Read the model definition and answer for the solid it produces. Units are mm, in the model's axes. Face numbers are marked on the shaded views. A direction names the side the tool comes from. Coordinates: 2 decimals unless noted, no trailing zeros. Order: outer loops, then holes, each group sorted by start corner. A loop starts at its lowest first (then second) coordinate and runs counter-clockwise, first axis right, second up. Notation, with made-up numbers: M 53,-38.75 L 67,-38.75 A33 ccw 67,-6.75 Z; hole C -11.75,-9 d3. An arc over 180 degrees is marked long. Use a Markdown table: item, result. Add a question column.
1) Find section A-A on x = 62. Write down the section's boundary in (y, z), plus the area to 3 significant figures.
2) For the marked faces 1 and 2, determine the directions among +Z, -Z, +X, -X, +Y, -Y from which every point of the face is accessible in a straight line to the end or side of a thin tool.
3) Find section B-B on y = 5. Count the separate pieces of the cut face and the enclosed holes in it, plus the area to 3 significant figures.
4) Find section D-D on y = 69.5. Write down the section's boundary in (x, z).
5) Find the intervals of material crossed by probe 1 along Y at (x, z) = (53, 17); probe 2 along X at (y, z) = (6, 10.5); probe 3 along Z at (x, y) = (73, 27.5), in increasing order. Write a range as [from, to].
6) Find section C-C on z = 126. Write down the section's boundary in (x, y), plus the area to 3 significant figures.
7) Each of these flat-tipped pins is pushed along its axis until it touches: pin 1 Ø6 at (x, z) = (59, 127) entering from +Y; pin 2 Ø5.5 at (y, z) = (22, -18.5) entering from +X; pin 3 Ø15.5 at (x, z) = (88, 159) entering from +Y. Where does it stop, or does it pass through?
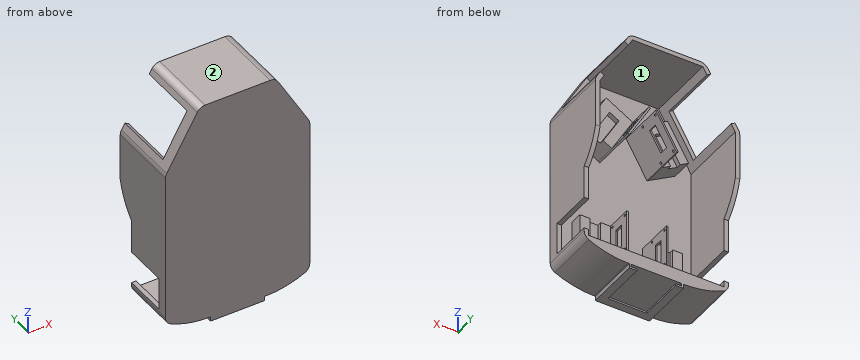
from build123d import *

# Parameters (mm, degrees)
BOSS_EXTRUDE1_DEPTH  = 80
BOSS_EXTRUDE2_DEPTH  = 2
SKETCH9_W            = 34
SKETCH9_H            = 46.5
BOSS_EXTRUDE3_DEPTH  = 13.75
SKETCH13_W           = 46.5
SKETCH13_H           = 42.25
BOSS_EXTRUDE7_DEPTH  = 2
SKETCH14_R           = 1.25
SKETCH14_W           = 25
SKETCH14_H           = 10
CUT_EXTRUDE1_DEPTH   = 2
SKETCH15_W           = 12
SKETCH15_H           = 35
CUT_EXTRUDE2_DEPTH   = 5
CUT_EXTRUDE3_DEPTH   = 298.215141228
FILLET5_R            = 10
SKETCH16_W           = 36
SKETCH16_H           = 48
CUT_EXTRUDE4_DEPTH   = 5
BOSS_EXTRUDE16_DEPTH = 23.75
SKETCH39_W           = 46.5
SKETCH39_H           = 52.25
BOSS_EXTRUDE17_DEPTH = 2
SKETCH40_R           = 1.25
SKETCH40_W           = 25
SKETCH40_H           = 10
CUT_EXTRUDE10_DEPTH  = 2
CUT_EXTRUDE11_DEPTH  = 5
SKETCH43_W           = 54
SKETCH43_H           = 67
CUT_EXTRUDE12_DEPTH  = 5
SKETCH44_W           = 150
SKETCH44_H           = 10
BOSS_EXTRUDE18_DEPTH = 60
SKETCH45_W           = 60
SKETCH45_H           = 60
BOSS_EXTRUDE19_DEPTH = 5
FILLET8_R            = 10
FILLET9_R            = 100
CUT_EXTRUDE13_DEPTH  = 51
SKETCH48_W           = 56
SKETCH48_H           = 3
CUT_EXTRUDE14_DEPTH  = 7


with BuildPart() as part:
    # Sketch1 → Boss-Extrude1 (new body)
    with BuildSketch(Plane(origin=(0, 0, 0), x_dir=(1, 0, 0), z_dir=(0, 1, 0))):
        Polygon((-5, 5), (-5, -171.339745962), (33.113248654, -237.353829072), (116.886751346, -237.353829072), (155, -171.339745962), (155, 5), align=None)
        Polygon((0, 0), (0, -170), (36, -232.353829072), (114, -232.353829072), (150, -170), (150, 0), align=None, mode=Mode.SUBTRACT)
    extrude(amount=BOSS_EXTRUDE1_DEPTH)



with BuildPart() as body_2:
    # Sketch8 → Boss-Extrude2 (new body)
    with BuildSketch(Plane.XZ):
        Polygon((0, 0), (0, 170), (36, 232.353829072), (114, 232.353829072), (150, 170), (150, 0), align=None)
    extrude(amount=-BOSS_EXTRUDE2_DEPTH)


with BuildPart() as part_1:
    add(part.part)

    add(body_2.part)  # Boss-Extrude3 merges body 2
    # Sketch9 → Boss-Extrude3 (add)
    with BuildSketch(Plane(origin=(0, 2, 0), x_dir=(1, 0, 0), z_dir=(0, 1, 0))):
        with Locations((115, -37)):
            Rectangle(SKETCH9_W, SKETCH9_H)
    boss_extrude3 = extrude(amount=BOSS_EXTRUDE3_DEPTH)

    # Sketch13 → Boss-Extrude7 (add)
    with BuildSketch(Plane.ZY.offset(-98)):
        with Locations((37, 23.125)):
            Rectangle(SKETCH13_W, SKETCH13_H)
    boss_extrude7 = extrude(amount=BOSS_EXTRUDE7_DEPTH)

    # Sketch14 → Cut-Extrude1 (cut)
    with BuildSketch(Plane.ZY.offset(-96)):
        with Locations((17, 41)):
            Circle(SKETCH14_R)
        with Locations((57, 41)):
            Circle(SKETCH14_R)
        with Locations(Location((57, 19, 0), (0, 0, 180))):
            Circle(SKETCH14_R)
        with Locations(Location((17, 19, 0), (0, 0, 180))):
            Circle(SKETCH14_R)
        with Locations((37, 30)):
            Rectangle(SKETCH14_W, SKETCH14_H)
    cut_extrude1 = extrude(amount=-CUT_EXTRUDE1_DEPTH, mode=Mode.SUBTRACT)

    # Sketch15 → Cut-Extrude2 (cut)
    with BuildSketch(Plane(origin=(0, 15.75, 0), x_dir=(1, 0, 0), z_dir=(0, 1, 0))):
        with Locations((115, -42.75)):
            Rectangle(SKETCH15_W, SKETCH15_H)
    cut_extrude2 = extrude(amount=-CUT_EXTRUDE2_DEPTH, mode=Mode.SUBTRACT)

    # Sketch17 → Cut-Extrude3 (cut, through all)
    with BuildSketch(Plane(origin=(155, 0, 0), x_dir=(0, 0, -1), z_dir=(1, 0, 0))):
        with BuildLine():
            Line((5, 60), (-80, 60))
            ThreePointArc((-80, 60), (-96.561006469, 72.526691771), (-115.934560766, 80))
            Line((-115.934560766, 80), (5, 80))
            Line((5, 80), (5, 60))
        make_face()
    extrude(amount=-CUT_EXTRUDE3_DEPTH, mode=Mode.SUBTRACT)

    # Fillet5
    fillet5_edges = [part_1.edges().sort_by_distance(p)[0] for p in [
        (-5, 40, 171.339745962),
        (33.113248654, 40, 237.353829072),
        (116.886751346, 40, 237.353829072),
        (155, 40, 171.339745962),
    ]]
    fillet(fillet5_edges, radius=FILLET5_R)

    # Sketch16 → Cut-Extrude4 (cut)
    with BuildSketch(Plane.ZY.offset(-150)):
        with Locations((25, 36)):
            Rectangle(SKETCH16_W, SKETCH16_H)
    cut_extrude4 = extrude(amount=-CUT_EXTRUDE4_DEPTH, mode=Mode.SUBTRACT)

    # Sketch38 → Boss-Extrude16 (add)
    with BuildSketch(Plane(origin=(0, 2, 0), x_dir=(1, 0, 0), z_dir=(0, 1, 0))):
        Polygon((109.054491924, -200.919700329), (132.304491924, -160.649519053), (102.859628196, -143.649519053), (79.609628196, -183.919700329), align=None)
    boss_extrude16 = extrude(amount=BOSS_EXTRUDE16_DEPTH)

    # Sketch39 → Boss-Extrude17 (add)
    with BuildSketch(Plane(origin=(139.346787517, 0, 80.451905284), x_dir=(-0.4999999999999941, 0, 0.866025403784442), z_dir=(-0.8660254037844421, 0, -0.49999999999999417))):
        with Locations((96.224318643, 28.125)):
            Rectangle(SKETCH39_W, SKETCH39_H)
    boss_extrude17 = extrude(amount=BOSS_EXTRUDE17_DEPTH)

    # Sketch40 → Cut-Extrude10 (cut)
    with BuildSketch(Plane(origin=(137.61473671, 0, 79.451905284), x_dir=(-0.4999999999999936, 0, 0.8660254037844424), z_dir=(-0.8660254037844424, 0, -0.4999999999999936))):
        with Locations((76.224318643, 51)):
            Circle(SKETCH40_R)
        with Locations(Location((116.224318643, 51, 0), (0, 0, 180))):
            Circle(SKETCH40_R)
        with Locations((116.224318643, 29)):
            Circle(SKETCH40_R)
        with Locations(Location((76.224318643, 29, 0), (0, 0, 180))):
            Circle(SKETCH40_R)
        with Locations((96.224318643, 40)):
            Rectangle(SKETCH40_W, SKETCH40_H)
    cut_extrude10 = extrude(amount=-CUT_EXTRUDE10_DEPTH, mode=Mode.SUBTRACT)

    # Sketch42 → Cut-Extrude11 (cut)
    with BuildSketch(Plane(origin=(0, 25.75, 0), x_dir=(1, 0, 0), z_dir=(0, 1, 0))):
        Polygon((105.278212483, -185.460408185), (122.778212483, -155.149519053), (112.385907637, -149.149519053), (94.885907637, -179.460408185), align=None)
    cut_extrude11 = extrude(amount=-CUT_EXTRUDE11_DEPTH, mode=Mode.SUBTRACT)

    # Sketch43 → Cut-Extrude12 (cut)
    with BuildSketch(Plane(origin=(186.112159322, 0, 107.451905284), x_dir=(-0.5000000000000009, 0, 0.8660254037844383), z_dir=(-0.8660254037844382, 0, -0.5000000000000008))):
        with Locations((108.224318643, 46.5)):
            Rectangle(SKETCH43_W, SKETCH43_H)
    cut_extrude12 = extrude(amount=-CUT_EXTRUDE12_DEPTH, mode=Mode.SUBTRACT)

    # Mirror1: Boss-Extrude3, Boss-Extrude7, Cut-Extrude1, Cut-Extrude2, Cut-Extrude4, Boss-Extrude16, Boss-Extrude17, Cut-Extrude10, Cut-Extrude11, Cut-Extrude12 across plane
    add(boss_extrude3.mirror(Plane.ZY.offset(-75)))
    add(boss_extrude7.mirror(Plane.ZY.offset(-75)))
    add(cut_extrude1.mirror(Plane.ZY.offset(-75)), mode=Mode.SUBTRACT)
    add(cut_extrude2.mirror(Plane.ZY.offset(-75)), mode=Mode.SUBTRACT)
    add(cut_extrude4.mirror(Plane.ZY.offset(-75)), mode=Mode.SUBTRACT)
    add(boss_extrude16.mirror(Plane.ZY.offset(-75)))
    add(boss_extrude17.mirror(Plane.ZY.offset(-75)))
    add(cut_extrude10.mirror(Plane.ZY.offset(-75)), mode=Mode.SUBTRACT)
    add(cut_extrude11.mirror(Plane.ZY.offset(-75)), mode=Mode.SUBTRACT)
    add(cut_extrude12.mirror(Plane.ZY.offset(-75)), mode=Mode.SUBTRACT)

    # Sketch44 → Boss-Extrude18 (add)
    with BuildSketch(Plane(origin=(0, 60, 0), x_dir=(1, 0, 0), z_dir=(0, 1, 0))):
        with Locations((75, 10)):
            Rectangle(SKETCH44_W, SKETCH44_H)
    extrude(amount=-BOSS_EXTRUDE18_DEPTH)

    # Sketch45 → Boss-Extrude19 (add)
    with BuildSketch(Plane(origin=(0, 0, -15), x_dir=(-1, 0, 0), z_dir=(0, 0, -1))):
        with Locations((-75, 30)):
            Rectangle(SKETCH45_W, SKETCH45_H)
    extrude(amount=BOSS_EXTRUDE19_DEPTH)

    # Fillet8
    # the kernel refuses this fillet: 10 mm, written as the material it takes off along each edge
    with BuildSketch(Plane(origin=(155, -21.650635095, -5), x_dir=(0, 0, 1), z_dir=(0, 1, 0))) as fillet8_piece_1:
        with BuildLine():
            CenterArc((8.660254038, -10), FILLET8_R, 90, 60)
            Line((0, -5), (-0.173205081, -4.9))
            ThreePointArc((-0.173205081, -4.9), (-0.2, -2.5), (-0.2, 0))
            Line((-0.2, 0), (0, 0.2))
            Line((0, 0.2), (8.660254038, 0.2))
            Line((8.660254038, 0.2), (8.660254038, 0))
        make_face()
    extrude(amount=103.301270189, mode=Mode.SUBTRACT)
    with BuildSketch(Plane(origin=(-5, -21.650635095, -5), x_dir=(0, 0, 1), z_dir=(0, 1, 0))) as fillet8_piece_2:
        with BuildLine():
            CenterArc((8.660254038, 10), FILLET8_R, 210, 60)
            Line((0, 5), (-0.173205081, 4.9))
            ThreePointArc((-0.173205081, 4.9), (-0.2, 2.5), (-0.2, 0))
            Line((-0.2, 0), (0, -0.2))
            Line((0, -0.2), (8.660254038, -0.2))
            Line((8.660254038, -0.2), (8.660254038, 0))
        make_face()
    extrude(amount=103.301270189, mode=Mode.SUBTRACT)

    # Fillet9
    # the kernel refuses this fillet: 100 mm, written as the material it takes off along each edge
    with BuildSketch(Plane(origin=(150, 168.972473589, -15), x_dir=(-1, 0, 0), z_dir=(0, -1, 0))) as fillet9_piece_1:
        with BuildLine():
            CenterArc((43.588989435, -100), FILLET9_R, 90, 25.841932763)
            Line((0, -10), (0, 0))
            Line((0, 0), (43.588989435, 0))
        make_face()
    extrude(amount=277.944947177, mode=Mode.SUBTRACT)
    with BuildSketch(Plane(origin=(0, 168.972473589, -15), x_dir=(0, 0, 1), z_dir=(0, -1, 0))) as fillet9_piece_2:
        with BuildLine():
            CenterArc((100, -43.588989435), FILLET9_R, 154.158067237, 25.841932763)
            Line((0, -43.588989435), (0, 0))
            Line((0, 0), (10, 0))
        make_face()
    extrude(amount=277.944947177, mode=Mode.SUBTRACT)

    # Sketch46 → Cut-Extrude13 (cut)
    with BuildSketch(Plane(origin=(0, 60, 0), x_dir=(1, 0, 0), z_dir=(0, 1, 0))):
        Polygon((53.5, 20), (96.5, 20), (96.5, 18), (103, 18), (103, 15), (47, 15), (47, 18), (53.5, 18), align=None)
    extrude(amount=-CUT_EXTRUDE13_DEPTH, mode=Mode.SUBTRACT)

    # Sketch48 → Cut-Extrude14 (cut)
    with BuildSketch(Plane(origin=(0, 9, 0), x_dir=(1, 0, 0), z_dir=(0, 1, 0))):
        with Locations((75, 16.5)):
            Rectangle(SKETCH48_W, SKETCH48_H)
    extrude(amount=-CUT_EXTRUDE14_DEPTH, mode=Mode.SUBTRACT)


solid = part_1.part
Check result:
| question | item | result |
|---|---|---|
| 1 | outline | M 0,-20 L 9,-20 L 9,-18 L 2,-18 L 2,-15 L 60,-15 L 60,0 L 2,0 L 2,165.39 L 35,165.39 L 35,169.39 L 25.75,169.39 L 25.75,188.76 L 2,188.76 L 2,232.35 L 80,232.35 L 80,237.35 L 0,237.35 Z; M 45,165.39 L 54.25,165.39 L 54.25,169.39 L 45,169.39 Z |
| 1 | area | 2,420 mm2 |
| 2 | face 1 | +Y |
| 2 | face 2 | +Z, +X, -X, +Y, -Y |
| 3 | separate pieces | 5 |
| 3 | enclosed holes | 2 |
| 3 | area | 11,700 mm2 |
| 4 | outline | M -5,91.59 L 0,91.59 L 0,170 L 4.5,177.79 L 0.17,180.29 L -3.66,173.66 A10 ccw -5,168.66 Z; M 27.17,227.06 L 31.5,224.56 L 36,232.35 L 114,232.35 L 118.5,224.56 L 122.83,227.06 L 119.77,232.35 A10 ccw 111.11,237.35 L 38.89,237.35 A10 ccw 30.23,232.35 Z; M 145.5,177.79 L 150,170 L 150,91.59 L 155,91.59 L 155,168.66 A10 ccw 153.66,173.66 L 149.83,180.29 Z |
| 5 | probe 1 | y = [0, 17.75], [20.25, 39.75], [42.25, 44.25] |
| 5 | probe 2 | x = [-5, 0], [150, 155] |
| 5 | probe 3 | z = [-15, 0], [232.35, 237.35] |
| 6 | outline | M -5,0 L 155,0 L 155,80 L 150,80 L 150,2 L 0,2 L 0,80 L -5,80 Z |
| 6 | area | 1,100 mm2 |
| 7 | pin 1 | stops at y = 2 |
| 7 | pin 2 | stops at x = 105 |
| 7 | pin 3 | stops at y = 54.25 |
